```python
from build123d import *

# Parameters (mm, degrees)
SKETCH1_R           = 4.5
BOSS_EXTRUDE1_DEPTH = 8.2
SKETCH2_R           = 11
BOSS_EXTRUDE2_DEPTH = 5
SKETCH3_R           = 1
CUT_EXTRUDE1_DEPTH  = 21.40196069
SKETCH4_R           = 1.5
CUT_EXTRUDE2_DEPTH  = 21.40196069
CHAMFER1_SIZE       = 1.5
CHAMFER1_SIZE2      = 0.866025404


with BuildPart() as part:
    # Sketch1 → Boss-Extrude1 (new body)
    with BuildSketch(Plane(origin=(0, 0, 0), x_dir=(1, 0, 0), z_dir=(0, 1, 0))):
        with Locations(Location((0, 0, 0), (0, 0, 270))):
            Circle(SKETCH1_R)
        with BuildLine():
            Line((-1.9, 1.953362486), (-1.9, -1.953362486))
            ThreePointArc((-1.9, -1.953362486), (0, -2.725), (1.9, -1.953362486))
            Line((1.9, -1.953362486), (1.9, 1.953362486))
            ThreePointArc((1.9, 1.953362486), (0, 2.725), (-1.9, 1.953362486))
        make_face(mode=Mode.SUBTRACT)
    extrude(amount=BOSS_EXTRUDE1_DEPTH)

    # Sketch2 → Boss-Extrude2 (add)
    with BuildSketch(Plane.XZ):
        with Locations(Location((0, 0, 0), (0, 0, 270))):
            Circle(SKETCH2_R)
    extrude(amount=BOSS_EXTRUDE2_DEPTH)

    # Sketch3 → Cut-Extrude1 (cut, through all)
    with BuildSketch(Plane.XZ.offset(5)):
        with Locations(Location((0, 0, 0), (0, 0, 270))):
            Circle(SKETCH3_R)
    extrude(amount=-CUT_EXTRUDE1_DEPTH, mode=Mode.SUBTRACT)

    # Sketch4 → Cut-Extrude2 (cut, through all)
    with BuildSketch(Plane.XZ.offset(5)):
        with Locations(Location((0, 8, 0), (0, 0, 270))):
            Circle(SKETCH4_R)
        with Locations(Location((-8, 0, 0), (0, 0, 270))):
            Circle(SKETCH4_R)
        with Locations(Location((0, -8, 0), (0, 0, 270))):
            Circle(SKETCH4_R)
        with Locations(Location((8, 0, 0), (0, 0, 270))):
            Circle(SKETCH4_R)
    extrude(amount=-CUT_EXTRUDE2_DEPTH, mode=Mode.SUBTRACT)

    # Chamfer1
    chamfer1_edges = [part.edges().sort_by_distance(p)[0] for p in [
        (0, -5, 1),
    ]]
    chamfer1_side = [part.faces().sort_by_distance(p)[0] for p in [
        (0, -5, 10.688873016),
    ]]
    chamfer(chamfer1_edges, length=CHAMFER1_SIZE, length2=CHAMFER1_SIZE2, reference=chamfer1_side[0])


solid = part.part
```
For this review, take the finished solid that the model builds, in its own axes (mm). A direction names the side the tool comes from. Coordinates: 2 decimals unless noted, no trailing zeros. Write each loop counter-clockwise with the first axis right and the second up, starting at its lowest first coordinate (ties: lowest second). Pieces come first, ordered by that corner, then holes.
(1) For pin 1 Ø2.5 at (x, z) = (-8, 0) entering from +Y; pin 2 Ø1.5 at (x, y) = (4, -1) entering from -Z; pin 3 Ø3.5 at (x, z) = (0, -8) entering from +Y; pin 4 Ø1.2 at (y, z) = (5, 0) entering from +X, all flat-tipped, find the tip position at first contact; note any pin that passes through.
(2) The part is to be moulded in two halves that separate along X. For faces 3 (the face through (1.352, 4.043, 4.292)), 4 (the face through (3, -5, 0)), 5 (the face through (0.07, -2.54, 9.5)), say which applies: +X half, -X half, draft (parallel to the pull), parting line (faces both ways), or undercut.
(3) Tool access review of faces 1 (the face through (2.1, 8.2, -0.1)), 2 (the face through (1.9, 4, 0)): name each direction out of +Z, -Z, +X, -X, +Y, -Y from which nothing blocks a thin tool from reaching the whole face with its end or side.
(4) Add section D-D on x = -8. Give the boundary of the cut face in (y, z), then the cut area to 3 significant figures.
(5) Wall thickness on probe 1 along X at (y, z) = (-3.6, 0); probe 2 along X at (y, z) = (7.5, 0); probe 3 along Y at (x, z) = (7.25, -3): over which ranges is each line inside the solid? List them lowest first.
(6) Add section B-B on z = 8. Give the boundary of the cut face in (x, y).
(7) Add section A-A on x = 0. Give the boundary of the cut face in (y, z) (3 decimals), then the cut area to 3 significant figures.
(8) Add section C-C on y = -1.5. Give the boundary of the cut face in (x, z).
Answer sheet:
1. pin 1: passes through
1. pin 2: stops at z = -10.51
1. pin 3: stops at y = 0
1. pin 4: stops at x = 4.5
2. face 3: parting line
2. face 4: draft
2. face 5: undercut
3. face 1: +Z, -Z, +X, -X, +Y
3. face 2: +Y
4. outline: (-5, -7.55) - (0, -7.55) - (0, -1.5) - (-5, -1.5) - close; (-5, 1.5) - (0, 1.5) - (0, 7.55) - (-5, 7.55) - close
4. area: 60.5 mm2
5. probe 1: x = -11 to -9.5, -6.5 to -1, 1 to 6.5, 9.5 to 11
5. probe 2: x = -4.5 to -1.9, 1.9 to 4.5
5. probe 3: y = -5 to 0
6. outline: (-7.55, -5) - (-1.5, -5) - (-1.5, 0) - (-7.55, 0) - close; (1.5, -5) - (7.55, -5) - (7.55, 0) - (1.5, 0) - close
7. outline: (-5, -11) - (0, -11) - (0, -9.5) - (-5, -9.5) - close; (-5, -6.5) - (0, -6.5) - (0, -4.5) - (8.2, -4.5) - (8.2, -2.725) - (0, -2.725) - (0, -1) - (-4.134, -1) - (-5, -2.5) - close; (-5, 2.5) - (-4.134, 1) - (0, 1) - (0, 2.725) - (8.2, 2.725) - (8.2, 4.5) - (0, 4.5) - (0, 6.5) - (-5, 6.5) - close; (-5, 9.5) - (0, 9.5) - (0, 11) - (-5, 11) - close
7. area: 97.8 mm2
8. outline: circle Ø22 at (0, 0); hole circle Ø3 at (-8, 0); hole circle Ø3 at (0, -8); hole circle Ø3 at (0, 8); hole circle Ø2 at (0, 0); hole circle Ø3 at (8, 0)
